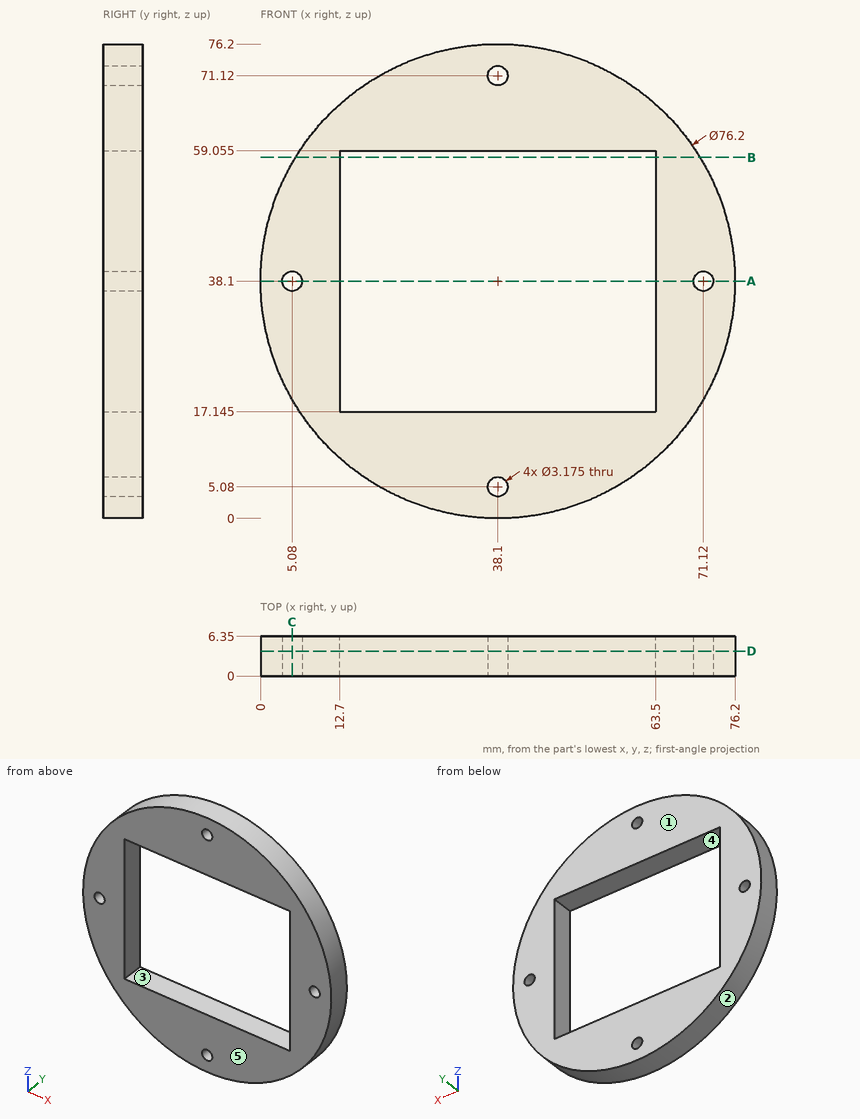
Study the drawing (mm; zero at the part's minimum x, y, z) and answer. A direction names the side the tool comes from. Coordinates: 2 decimals unless noted, no trailing zeros. Loops run counter-clockwise (first coordinate to the right, second up) from the corner with the lowest first, then second, coordinate; pieces in that order, holes last. Notation, with made-up numbers: (-38.5, -12) -> (-18.5, -12) arc R18 cw to (-18.5, 23) -> close; hole circle Ø1 at (73, -40). An arc over 180 degrees is marked (long way). Answer in a Markdown table with one row per item. Add a question column.
1. Flat-ended cylindrical pins translate along their axes: P1, Ø1.9, axis at y = 3.5, z = 43.5, coming from the +X side; P2, Ø3, axis at x = 34, y = 4, coming from the +Z side. Find the tip coordinate at first contact, or state that the pin passes through.
2. The part is cut by section C-C, the plane x = 5.08. Write down the section's boundary in (y, z), then the cut area to 3 significant figures.
3. Determine the mould class of the marked faces 1, 2 and 3 for opening direction X: +X half, -X half, draft (parallel to the pull), parting line (faces both ways), or undercut.
4. For the marked faces 4 and 5, determine the directions among +Z, -Z, +X, -X, +Y, -Y from which every point of the face is accessible in a straight line to the end or side of a thin tool.
5. Consider line 1 (X direction, y = 4, z = 38.1); line 2 (X direction, y = 5.25, z = 37); line 3 (Z direction, x = 17, y = 2) (3 decimals). Determine where each line is inside the solid, lowest interval first. Write a range as [from, to].
6. The part is cut by section B-B, the plane z = 58. Write down the section's boundary in (x, y).
7. The part is cut by section A-A, the plane z = 38.1. Write down the section's boundary in (x, y).
8. The part is cut by section D-D, the plane y = 4. Write down the section's boundary in (x, z) (1 decimal).
Answer below:
| question | item | result |
|---|---|---|
| 1 | P1 | x = 75.94 |
| 1 | P2 | z = 76.11 |
| 2 | outline | (0, 19.09) -> (6.35, 19.09) -> (6.35, 36.51) -> (0, 36.51) -> close; (0, 39.69) -> (6.35, 39.69) -> (6.35, 57.11) -> (0, 57.11) -> close |
| 2 | area | 221 mm2 |
| 3 | face 1 | draft |
| 3 | face 2 | parting line |
| 3 | face 3 | undercut |
| 4 | face 4 | +Y, -Y |
| 4 | face 5 | +Z, -Z, +X, -X, -Y |
| 5 | line 1 | [0, 3.49], [6.67, 12.7], [63.5, 69.53], [72.71, 76.2] |
| 5 | line 2 | [0.02, 3.94], [6.22, 12.7], [63.5, 69.98], [72.26, 76.18] |
| 5 | line 3 | [6.376, 17.145], [59.055, 69.824] |
| 6 | outline | (5.61, 0) -> (12.7, 0) -> (12.7, 6.35) -> (5.61, 6.35) -> close; (63.5, 0) -> (70.59, 0) -> (70.59, 6.35) -> (63.5, 6.35) -> close |
| 7 | outline | (0, 0) -> (3.49, 0) -> (3.49, 6.35) -> (0, 6.35) -> close; (6.67, 0) -> (12.7, 0) -> (12.7, 6.35) -> (6.67, 6.35) -> close; (63.5, 0) -> (69.53, 0) -> (69.53, 6.35) -> (63.5, 6.35) -> close; (72.71, 0) -> (76.2, 0) -> (76.2, 6.35) -> (72.71, 6.35) -> close |
| 8 | outline | circle Ø76.2 at (38.1, 38.1); hole circle Ø3.2 at (5.1, 38.1); hole (12.7, 17.1) -> (63.5, 17.1) -> (63.5, 59.1) -> (12.7, 59.1) -> close; hole circle Ø3.2 at (38.1, 5.1); hole circle Ø3.2 at (38.1, 71.1); hole circle Ø3.2 at (71.1, 38.1) |
